```python
from build123d import *

# Parameters (mm, degrees)
CROQUIS3_W              = 25
CROQUIS3_H              = 35
SALIENTE_EXTRUIR2_DEPTH = 4
CROQUIS5_W              = 25
CROQUIS5_H              = 17.5
SALIENTE_EXTRUIR3_DEPTH = 2
CROQUIS7_W              = 25
CROQUIS7_H              = 10
SALIENTE_EXTRUIR5_DEPTH = 55
CROQUIS8_R              = 2.5
CORTAR_EXTRUIR1_DEPTH   = 55
SALIENTE_EXTRUIR6_DEPTH = 25
CROQUIS9_R              = 5.1
CORTAR_EXTRUIR3_DEPTH   = 4
CROQUIS11_R             = 2
CORTAR_EXTRUIR4_DEPTH   = 20
CROQUIS12_R             = 5.1
CORTAR_EXTRUIR5_DEPTH   = 45


with BuildPart() as part:
    # Croquis3 → Saliente-Extruir2 (new body)
    with BuildSketch(Plane(origin=(0, 0, 0), x_dir=(0, 0, -1), z_dir=(1, 0, 0))):
        with Locations((4.326923077, 2.8125)):
            Rectangle(CROQUIS3_W, CROQUIS3_H)
    extrude(amount=SALIENTE_EXTRUIR2_DEPTH)

    # Croquis5 → Saliente-Extruir3 (add)
    with BuildSketch(Plane(origin=(4, 0, 0), x_dir=(0, 0, -1), z_dir=(1, 0, 0))):
        with Locations((4.326923077, 11.5625)):
            Rectangle(CROQUIS5_W, CROQUIS5_H)
    extrude(amount=SALIENTE_EXTRUIR3_DEPTH)

    # Croquis7 → Saliente-Extruir5 (add)
    with BuildSketch(Plane(origin=(4, 0, 0), x_dir=(0, 0, -1), z_dir=(1, 0, 0))):
        with Locations((4.326923077, -2.1875)):
            Rectangle(CROQUIS7_W, CROQUIS7_H)
    extrude(amount=SALIENTE_EXTRUIR5_DEPTH)

    # Croquis8 → Cortar-Extruir1 (cut)
    with BuildSketch(Plane(origin=(6, 0, 0), x_dir=(0, 0, -1), z_dir=(1, 0, 0))):
        with Locations((4.326923077, 15.3125)):
            Circle(CROQUIS8_R)
        with Locations((4.326923077, 7.8125)):
            Circle(CROQUIS8_R)
    extrude(amount=-CORTAR_EXTRUIR1_DEPTH, mode=Mode.SUBTRACT)

    # Croquis10 → Saliente-Extruir6 (add, through all)
    with BuildSketch(Plane.XY.offset(8.173076923)):
        Polygon((4, -14.6875), (59, -7.1875), (4, -7.1875), align=None)
    extrude(amount=-SALIENTE_EXTRUIR6_DEPTH)

    # Croquis9 → Cortar-Extruir3 (cut)
    with BuildSketch(Plane(origin=(0, 2.8125, 0), x_dir=(1, 0, 0), z_dir=(0, 1, 0))):
        with Locations(Location((25, 4.326923077, 0), (0, 0, 270))):
            Circle(CROQUIS9_R)
    extrude(amount=-CORTAR_EXTRUIR3_DEPTH, mode=Mode.SUBTRACT)

    # Croquis11 → Cortar-Extruir4 (cut)
    with BuildSketch(Plane(origin=(59, 0, 0), x_dir=(0, 0, -1), z_dir=(1, 0, 0))):
        with Locations((-1.923076923, -2.1875)):
            Circle(CROQUIS11_R)
        with Locations((10.576923077, -2.1875)):
            Circle(CROQUIS11_R)
    extrude(amount=-CORTAR_EXTRUIR4_DEPTH, mode=Mode.SUBTRACT)

    # Croquis12 → Cortar-Extruir5 (cut)
    with BuildSketch(Plane(origin=(0, -1.1875, 0), x_dir=(1, 0, 0), z_dir=(0, 1, 0))):
        with Locations(Location((25, 4.326923077, 0), (0, 0, 270))):
            Circle(CROQUIS12_R)
    extrude(amount=-CORTAR_EXTRUIR5_DEPTH, mode=Mode.SUBTRACT)


solid = part.part
```
CAD build for the part. Positions are in the model's coordinates, mm. A direction names the side the tool comes from. Coordinates: 2 decimals unless noted, no trailing zeros. Order: outer loops, then holes, each group sorted by start corner. A loop starts at its lowest first (then second) coordinate and runs counter-clockwise, first axis right, second up.
(1) Drill centre lines: L1, parallel to Z at x = 25, y = -8; L2, parallel to X at y = 6, z = -9.5; L3, parallel to Y at x = 20, z = -11.5. Where is each one in solid material? Low to high.
Solution:
L1: z = -16.83 to -9.43, 0.77 to 8.17
L2: x = 0 to 6
L3: y = -12.51 to 2.81
(2) Saw through at A-A, the plane x = 26.5. Write the cut outline in (y, z).
Solution:
outline: (-11.62, -16.83) - (2.81, -16.83) - (2.81, -9.2) - (-11.62, -9.2) - close; (-11.62, 0.55) - (2.81, 0.55) - (2.81, 8.17) - (-11.62, 8.17) - close
(3) Saw through at D-D, the plane z = -15. Write the cut outline in (x, y), and give its area (3 significant figures).
Solution:
outline: (0, -14.69) - (4, -14.69) - (59, -7.19) - (59, 2.81) - (6, 2.81) - (6, 20.31) - (0, 20.31) - close
area: 931 mm2
(4) Saw through at C-C, the plane y = -1.5. Write the cut outline in (x, z), and give its area (3 significant figures).
Solution:
outline: (0, -16.83) - (59, -16.83) - (59, -12.46) - (39, -12.46) - (39, -8.7) - (59, -8.7) - (59, 0.04) - (39, 0.04) - (39, 3.8) - (59, 3.8) - (59, 8.17) - (0, 8.17) - close; hole circle Ø10.2 at (25, -4.33)
area: 1,240 mm2
(5) Saw through at B-B, the plane z = -6. Write the cut outline in (x, y), and give its area (3 significant figures).
Solution:
outline: (0, -14.69) - (4, -14.69) - (20.18, -12.48) - (20.18, 2.81) - (6, 2.81) - (6, 5.95) - (0, 5.95) - close; (0, 9.67) - (6, 9.67) - (6, 13.45) - (0, 13.45) - close; (0, 17.17) - (6, 17.17) - (6, 20.31) - (0, 20.31) - close; (29.82, -11.17) - (59, -7.19) - (59, 2.81) - (29.82, 2.81) - close
area: 746 mm2
(6) Pin check, flat tips, straight feed: pin 1 Ø13.5 at (x, z) = (25, -4.33) entering from +Y; pin 2 Ø5 at (y, z) = (-2.19, -10.58) entering from +X; pin 3 Ø4 at (y, z) = (6.5, -3.5) entering from +X; pin 4 Ø2 at (y, z) = (-2, 1) entering from +X. Stop position of each tip, or through.
Solution:
pin 1: stops at y = 2.81
pin 2: stops at x = 59
pin 3: stops at x = 6
pin 4: stops at x = 39
(7) Mould opens along Y. For faces 1 (the face through (3.042, 5.372, -3.785)), 2 (the face through (31.12, -10.99, -4.15)), 3 (the face through (20.02, -4.75, -5.43)) say: released by +Y, released by -Y, zero draft, split by the parting line, or undercut.
Solution:
face 1: undercut
face 2: released by -Y
face 3: zero draft
(8) Which spindle directions (+Z, -Z, +X, -X, +Y, -Y) get a long thin tool onto all of the face, cutting with end or side? Do faces 4 (the face through (6, 12, -4)), 5 (the face through (49.14, -1.587, -12.485)), 6 (the face through (3.042, 13.791, -2.343)). Say none if no direction does.
Solution:
face 4: +Z, -Z, +X, +Y
face 5: +X
face 6: +X, -X
